CAD build for the part. Positions are in the model's coordinates, mm. Give positions to 0.01 mm unless a question says otherwise; leave off trailing zeros. Write each loop counter-clockwise with the first axis right and the second up, starting at its lowest first coordinate (ties: lowest second). Pieces come first, ordered by that corner, then holes. Notation, with made-up numbers: (88.5, 10.25) -> (94.5, 10.25) arc R30 cw to (94.5, 41.25) -> close; hole circle Ø2 at (2.5, 76). An arc over 180 degrees is marked (long way). Answer in a Markdown table with one row per item. Add a question column.
```python
from build123d import *

# Parameters (mm, degrees)
SKETCH1_R               = 32.5
SKETCH1_W               = 6
SKETCH1_H               = 6
SKETCH1_W_2             = 27
SKETCH1_H_2             = 54
BOSS_EXTRUDE1_DEPTH     = 6
CUT_EXTRUDE2_DEPTH      = 47.351914739
CUT_EXTRUDE2_DEPTH_BACK = 47.351914739
SKETCH2_W               = 5
SKETCH2_H               = 5


with BuildPart() as part:
    # Sketch1 → Boss-Extrude1 (new body)
    with BuildSketch(Plane(origin=(0, 0, 0), x_dir=(1, 0, 0), z_dir=(0, 1, 0))):
        with Locations(Location((0, 0, 0), (0, 0, 270))):
            Circle(SKETCH1_R)
        with Locations((-20, 0)):
            Rectangle(SKETCH1_W, SKETCH1_H, mode=Mode.SUBTRACT)
        Rectangle(SKETCH1_W_2, SKETCH1_H_2, mode=Mode.SUBTRACT)
        with Locations((20, 0)):
            Rectangle(SKETCH1_W, SKETCH1_H, mode=Mode.SUBTRACT)
    extrude(amount=BOSS_EXTRUDE1_DEPTH)

    # Sketch2 → Cut-Extrude2 (cut, two sides: drawn at the far end of the back side and taken through both)
    with BuildSketch(Plane(origin=(0, 0, 0), x_dir=(1, 0, 0), z_dir=(0, 1, 0)).offset(-CUT_EXTRUDE2_DEPTH_BACK)):
        with Locations((-20, 13.5)):
            Rectangle(SKETCH2_W, SKETCH2_H)
        with Locations((-20, -13.5)):
            Rectangle(SKETCH2_W, SKETCH2_H)
        with Locations((20, -13.5)):
            Rectangle(SKETCH2_W, SKETCH2_H)
        with Locations((20, 13.5)):
            Rectangle(SKETCH2_W, SKETCH2_H)
    extrude(amount=CUT_EXTRUDE2_DEPTH + CUT_EXTRUDE2_DEPTH_BACK, mode=Mode.SUBTRACT)


solid = part.part
```
Item 1: Drop flat-ended pins along their axis: pin 1 Ø2 at (x, y) = (-25, 4.5) entering from -Z; pin 2 Ø2.5 at (x, y) = (19, 2) entering from -Z; pin 3 Ø3 at (x, y) = (8, 4.5) entering from +Z. Give the stop position or say it passes through.
Item 2: Mould opens along X. For faces 1 (the face through (9.76, 2.96, 31)), 2 (the face through (-14, 0, 0)), 3 (the face through (20, 3, -11)) say: released by +X, released by -X, zero draft, split by the parting line, or undercut.
Item 3: Slice it at A-A, the plane y = 1.6. State how many separate pieces and enclosed holes the cut face has, then the cut area to 3 significant figures.
Item 4: Slice it at D-D, the plane x = -20. List the corners of the cut face in (y, z).
Item 5: Probe L1, parallel to X at y = 3.3, z = -12.5; L2, parallel to X at y = 5.25, z = -26.5; L3, parallel to X at y = 2.6, z = 19. List the from-to ranges inside material, lowest first. Write a range as from..to.
Item 6: Slice it at B-B, the plane x = 0. List the corners of the cut face in (y, z).
Item 7: Slice it at C-C, the plane z = -13. List the corners of the cut face in (x, y).
Answer key:
| question | item | result |
|---|---|---|
| 1 | pin 1 | stops at z = -21.91 |
| 1 | pin 2 | stops at z = -27.22 |
| 1 | pin 3 | stops at z = 31.84 |
| 2 | face 1 | split by the parting line |
| 2 | face 2 | zero draft |
| 2 | face 3 | undercut |
| 3 | separate pieces | 1 |
| 3 | enclosed holes | 7 |
| 3 | area | 1,690 mm² |
| 4 | outline | (0, -25.62) -> (6, -25.62) -> (6, -16) -> (0, -16) -> close; (0, -11) -> (6, -11) -> (6, -3) -> (0, -3) -> close; (0, 3) -> (6, 3) -> (6, 11) -> (0, 11) -> close; (0, 16) -> (6, 16) -> (6, 25.62) -> (0, 25.62) -> close |
| 5 | L1 | x = -30..-22.5, -17.5..-13.5, 13.5..17.5, 22.5..30 |
| 5 | L2 | x = -18.81..-13.5, 13.5..18.81 |
| 5 | L3 | x = -26.37..-13.5, 13.5..26.37 |
| 6 | outline | (0, -32.5) -> (6, -32.5) -> (6, -27) -> (0, -27) -> close; (0, 27) -> (6, 27) -> (6, 32.5) -> (0, 32.5) -> close |
| 7 | outline | (-29.79, 0) -> (-22.5, 0) -> (-22.5, 6) -> (-29.79, 6) -> close; (-17.5, 0) -> (-13.5, 0) -> (-13.5, 6) -> (-17.5, 6) -> close; (13.5, 0) -> (17.5, 0) -> (17.5, 6) -> (13.5, 6) -> close; (22.5, 0) -> (29.79, 0) -> (29.79, 6) -> (22.5, 6) -> close |
